Autodesk Inventor part; units mm, degrees
ref_plane "Work Plane1" through (31, 0, 0) normal (1, 0, 0) x (0, 1, 0)
ref_plane "XZ Plane" through (0, 0, 0) normal (0, 1, 0) x (-1, 0, 0)
ref_plane "XY Plane" through (0, 0, 0) normal (0, 0, 1) x (1, 0, 0)
sketch "Sketch2" plane through (0, 0, 0) normal (0, 0, 1) x (1, 0, 0)
  line L0 (-55, 0) -> (55, 0)
  line L1 (55, 0) -> (55, 116)
  arc A0 (55, 116) -> (-55, 116) centre (0, 116) ccw
  line L2 (-55, 116) -> (-55, 0)
  point P0 (0, 0)
  point P1 (0, 0)
  dimension "d0" = 55
  dimension "d1" = 116
extrude "Extrusion1" add sketch "Sketch2" along normal mid plane 1.5
sketch "Sketch3" plane through (0, 0, 0.75) normal (0, 0, 1) x (1, 0, 0)
  line L0 (-22.5, 14) -> (22.5, 14)
  line L1 (22.5, 14) -> (22.5, 40.9816)
  line L2 (-22.5, 40.9816) -> (-22.5, 14)
  arc A0 (22.5, 40.9816) -> (-22.5, 40.9816) centre (0, -20) ccw
  arc A1 (55, 116) -> (-55, 116) centre (0, 116) ccw
  line L3 (-55, 0) -> (55, 0)
  point P0 (0, 0)
  point P1 (0, 14)
  point P2 (0, 171)
  point P3 (0, 45)
  dimension "d4" = 65
  dimension "d5" = 45
  dimension "d6" = 14
  dimension "d7" = 31
extrude "Extrusion2" cut sketch "Sketch3" against normal up to surface (1.5 mm away)
sketch "Sketch4" plane through (0, 0, 0.75) normal (0, 0, 1) x (1, 0, 0)
  line L0 (-7.5, 63.5) -> (7.5, 63.5)
  line L1 (7.5, 63.5) -> (7.5, 78.5)
  line L2 (7.5, 78.5) -> (-7.5, 78.5)
  line L3 (-7.5, 78.5) -> (-7.5, 63.5)
  line L4 (-7.5, 153.5) -> (7.5, 153.5)
  line L5 (7.5, 153.5) -> (7.5, 168.5)
  line L6 (7.5, 168.5) -> (-7.5, 168.5)
  line L7 (-7.5, 168.5) -> (-7.5, 153.5)
  arc A0 (22.5, 40.9816) -> (-22.5, 40.9816) centre (0, -20) ccw
  arc A1 (55, 116) -> (-55, 116) centre (0, 116) ccw
  point P0 (0, 0)
  point P1 (0, 153.5)
  point P2 (0, 45)
  point P3 (0, 63.5)
  point P4 (0, 45)
  point P5 (7.5, 71)
  dimension "d10" = 15
  dimension "d11" = 15
  dimension "d12" = 15
  dimension "d13" = 15
  dimension "d14" = 37.5
  dimension "d15" = 37.5
extrude "Extrusion3" cut sketch "Sketch4" against normal up to surface (1.5 mm away)
sketch "Sketch6" plane through (55, 0, 0.75) normal (1, 0, 0) x (0, 0, -1)
  line L0 (0, 0) -> (0, 116)
  line L1 (1.5, 116) -> (0, 116)
  line L2 (1.5, 116) -> (1.5, 0)
  line L3 (0, 0) -> (1.5, 0)
  line L4 (0, -0.3907) -> (9.5, -0.3907)
  line L5 (9.5, -0.3907) -> (9.5, 116)
  line L6 (9.5, 116) -> (0, 116)
  line L7 (0, 116) -> (0, -0.3907)
  point P0 (0.75, 0)
  dimension "d18" = 9.5
extrude "Extrusion4" add sketch "Sketch6" against normal blind 1.5
sketch "Sketch7" plane through (55, -0.3907, 0.75) normal (1, 0, 0) x (0, 0, -1)
  line L0 (0, 0) -> (9.5, 0)
  line L1 (0, 116.3907) -> (0, 0)
  point P0 (0.75, 0.3907)
  point P1 (5, 109.5)
  point P2 (5, 84.5)
  point P3 (5, 59.5)
  point P4 (5, 34.5)
  point P5 (5, 9.5)
  dimension "d21" = 9.5
  dimension "d22" = 25
  dimension "d23" = 25
  dimension "d24" = 25
  dimension "d25" = 25
  dimension "d26" = 5
hole "Hole1" at (55, 109.1093, -4.25) at (55, 84.1093, -4.25) at (55, 59.1093, -4.25) at (55, 34.1093, -4.25) at (55, 9.1093, -4.25) direction (-1, 0, 0) diameter 3 depth 1.5
mirror "Mirror1" about plane through (0, 0, 0) normal (1, 0, 0) of "Extrusion4", "Hole1"
ref_plane "Work Plane1" through (31, 0, 0) normal (1, 0, 0) x (0, 1, 0)
sketch "Sketch8" plane through (31, 0, 0) normal (1, 0, 0) x (0, 1, 0)
  point P0 (0, 0)
sketch "Sketch9" plane through (31, 0, 0) normal (1, 0, 0) x (0, 1, 0)
  line L0 (40.9816, 0.75) -> (14, 0.75)
  line L1 (14, 0.75) -> (40.9816, 0.75)
  line L2 (34.6093, 0.75) -> (34.6093, 5.25)
  line L3 (34.6093, 5.25) -> (19.6093, 5.25)
  line L4 (19.6093, 5.25) -> (19.6093, 0.75)
  line L5 (-0.3907, -8.75) -> (-0.3907, 0.75)
  point P0 (0, 0)
  dimension "d35" = 20
  dimension "d36" = 15
  dimension "d37" = 4.5
extrude "Extrusion5" add sketch "Sketch9" along normal blind 6
sketch "Sketch10" plane through (31, 34.6093, 5.25) normal (0, 1, 0) x (1, 0, 0)
  line L0 (0, 4.5) -> (0, 0)
  line L1 (0, 0) -> (6, 0)
  line L2 (6, 4.5) -> (6, 0)
  line L3 (0, 4.5) -> (6, 4.5)
  arc A0 (0, 0) -> (6, 0) centre (3, 0) ccw
  point P0 (-31, 5.25)
extrude "Extrusion6" add sketch "Sketch10" against normal up to surface (15 mm away) contours L1 A0
sketch "Sketch11" plane through (31, 19.6093, 0.75) normal (0, -1, 0) x (1, 0, 0)
  arc A0 (6, 4.5) -> (0, 4.5) centre (3, 4.5) ccw
  point P0 (-31, -0.75)
  point P1 (3, 7.5)
hole "Hole2" at (34, 19.6093, 5.25) direction (0, 1, 0) diameter 3 depth 15
sketch "Sketch12" plane through (0, 0, 0.75) normal (0, 0, 1) x (1, 0, 0)
  circle A0 centre (-28.5, 23) radius 1.5
  line L0 (-22.5, 14) -> (-22.5, 40.9816)
  line L1 (-53.5, 0) -> (53.5, 0)
  point P0 (0, 0)
  dimension "d49" = 3
  dimension "d50" = 6
  dimension "d51" = 23
extrude "Extrusion7" cut sketch "Sketch12" against normal up to surface (1.5 mm away)
equation "\"d15\" = d14"
properties part number "1 part 07"
Work out the finished part from the listing and answer in its coordinate system (mm). A direction names the side the tool comes from. Round coordinates to 2 decimals unless told otherwise and drop trailing zeros. Write each loop counter-clockwise with the first axis right and the second up, starting at its lowest first coordinate (ties: lowest second). Pieces come first, ordered by that corner, then holes.
1) Which of the six approach directions +Z, -Z, +X, -X, +Y, -Y give full straight-line access (tool end or side, diameter ignored) to faces 1 (the face through (0, 45, 0)), 2 (the face through (34.6, 34.609, 3.6)), 3 (the face through (55, 57, -4)), 4 (the face through (34, 19.609, 3.6))?
2) A cutting plane is placed at A-A on x = 0. Determine the outline of the cut face in (y, z), and give its area (3 significant figures).
3) A cutting plane is placed at D-D on x = 46. Determine the outline of the cut face in (y, z).
4) Consider probe 1 along Y at (x, z) = (-53.8, -4.25); probe 2 along X at (y, z) = (31.75, 5.25); probe 3 along X at (y, z) = (66.5, -7.5). Determine where each line is inside the solid, lowest interval first.
5) A cutting plane is placed at B-B on x = -15. Determine the outline of the cut face in (y, z).
6) A cutting plane is placed at C-C on y = 132.5. Determine the outline of the cut face in (x, z).
7) Flat-ended cylindrical pins translate along their axes: P1, Ø4, axis at x = 34, z = 5.25, coming from the -Y side; P2, Ø1.6, axis at x = 3.5, z = 0, coming from the -Y side; P3, Ø8, axis at x = 15, y = 78, coming from the -Z side; P4, Ø3.5, axis at y = 34.11, z = -4.25, coming from the +X side. Find the tip coordinate at first contact, or state that the pin passes through.
8) Determine the mould class of faces 5 (the face through (31, 27, 3)), 6 (the face through (37, 27, 3)), 7 (the face through (-53.5, 59, -6)), 8 (the face through (33.93, 27.21, 8.25)) for opening direction X: pulls with the +X half, pulls with the -X half, needs draft (parallel to the pull), parting line crosses it, or undercut.
Entries:
1. face 1: +Z, -Z
1. face 2: +Z, +X, -X, +Y
1. face 3: +Z, -Z, +X, +Y, -Y
1. face 4: +Z, +X, -X, -Y
2. outline: (0, -0.75) - (14, -0.75) - (14, 0.75) - (0, 0.75) - close; (45, -0.75) - (63.5, -0.75) - (63.5, 0.75) - (45, 0.75) - close; (78.5, -0.75) - (153.5, -0.75) - (153.5, 0.75) - (78.5, 0.75) - close; (168.5, -0.75) - (171, -0.75) - (171, 0.75) - (168.5, 0.75) - close
2. area: 165 mm2
3. outline: (0, -0.75) - (146.15, -0.75) - (146.15, 0.75) - (0, 0.75) - close
4. probe 1: y = -0.39 to 7.61, 10.61 to 32.61, 35.61 to 57.61, 60.61 to 82.61, 85.61 to 107.61, 110.61 to 116
4. probe 2: x = 31 to 32.5, 35.5 to 37
4. probe 3: x = -55 to -53.5, 53.5 to 55
5. outline: (0, -0.75) - (14, -0.75) - (14, 0.75) - (0, 0.75) - close; (43.25, -0.75) - (168.92, -0.75) - (168.92, 0.75) - (43.25, 0.75) - close
6. outline: (-52.47, -0.75) - (52.47, -0.75) - (52.47, 0.75) - (-52.47, 0.75) - close
7. P1: stops at y = 19.61
7. P2: stops at y = 0
7. P3: stops at z = -0.75
7. P4: stops at x = 55
8. face 5: pulls with the -X half
8. face 6: pulls with the +X half
8. face 7: undercut
8. face 8: parting line crosses it
